from build123d import *

# Parameters (mm, degrees)
Y_KSEKLIK_EKSTR_ZYON1_DEPTH      = 370
Y_KSEKLIK_EKSTR_ZYON2_DEPTH      = 2
Y_KSEKLIK_EKSTR_ZYON2_DEPTH_BACK = 141
KES_EKSTR_ZYON1_DEPTH            = 141


with BuildPart() as part:
    # Çizim1 → Yükseklik-Ekstrüzyon1 (new body)
    with BuildSketch(Plane(origin=(0, 0, 0), x_dir=(0, -1, 0), z_dir=(-1, 0, 0))):
        Polygon((0, 0), (-4, 0), (-4, -4), (-3.5, -4), (-3.5, -0.5), (-0.5, -0.5), (-0.5, -13.15), (-3.5, -13.15), (-3.5, -9.65), (-4, -9.65), (-4, -13.65), (0, -13.65), align=None)
    extrude(amount=-Y_KSEKLIK_EKSTR_ZYON1_DEPTH)

    # Çizim3 → Yükseklik-Ekstrüzyon2 (add, two sides: drawn at the far end of the back side and taken through both)
    with BuildSketch(Plane.ZY.offset(-Y_KSEKLIK_EKSTR_ZYON2_DEPTH_BACK)):
        Polygon((-13.65, 0), (-13.65, 4), (-9.65, 4), (-9.65, 3.5), (-13.15, 3.5), (-13.15, 0.5), (-0.5, 0.5), (-0.5, 3.5), (-4, 3.5), (-4, 4), (0, 4), (0, 0), align=None)
    extrude(amount=Y_KSEKLIK_EKSTR_ZYON2_DEPTH + Y_KSEKLIK_EKSTR_ZYON2_DEPTH_BACK)

    # Çizim5 → Kes-Ekstrüzyon1 (cut)
    with BuildSketch(Plane.ZY.offset(2)):
        Polygon((-13.65, 4), (-13.65, 0), (0, 0), (0, 4), (-4, 4), (-4, 3.5), (-0.5, 3.5), (-0.5, 0.5), (-13.15, 0.5), (-13.15, 3.5), (-9.65, 3.5), (-9.65, 4), align=None)
    extrude(amount=-KES_EKSTR_ZYON1_DEPTH, mode=Mode.SUBTRACT)


solid = part.part
Verification items for the finished model (mm, model axes). A direction names the side the tool comes from. Coordinates: 2 decimals unless noted, no trailing zeros. Order: outer loops, then holes, each group sorted by start corner. A loop starts at its lowest first (then second) coordinate and runs counter-clockwise, first axis right, second up. Notation, with made-up numbers: M -18.5,14.5 L 31.5,14.5 A7 cw 31.5,25.5 Z; hole C 42.5,0.5 d5. An arc over 180 degrees is marked long. Write each question's results on one line, items separated by ' | '.
1) Gauge pin test, flat end, axial feed: pin 1 Ø3 at (x, z) = (255, -4.5) entering from +Y. Record the tip position at first contact, or that the pin passes through.
Solved:
pin 1: stops at y = 4
2) Scan lines: line 1 along Z through (x, y) = (211.5, 0.55); line 2 along Y through (x, z) = (243, -11.75); line 3 along Y through (x, z) = (215, -6.5). Record each from-to range of solid material in increasing order. Write a range as [from, to].
Solved:
line 1: z = [-13.65, -13.15], [-0.5, 0] | line 2: y = [0, 0.5], [3.5, 4] | line 3: y = [0, 0.5]
3) Section check C-C on z = -7.25. Record the cut outline in (x, y).
Solved:
outline: M 139,0 L 370,0 L 370,0.5 L 139,0.5 Z
4) Release check for a two-part mould opening along Y. For faces 3 (the face through (256, 0, -7)), 4 (the face through (256, 4, -12)), 5 (the face through (256, 3.5, -2)), 6 (the face through (370, 0.2, -6.3)) record: pulls with the +Y half, pulls with the -Y half, needs draft (parallel to the pull), parting line crosses it, or undercut.
Solved:
face 3: pulls with the -Y half | face 4: pulls with the +Y half | face 5: undercut | face 6: needs draft
5) Section check B-B on x = 296. Record the cut outline in (y, z).
Solved:
outline: M 0,-13.65 L 4,-13.65 L 4,-9.65 L 3.5,-9.65 L 3.5,-13.15 L 0.5,-13.15 L 0.5,-0.5 L 3.5,-0.5 L 3.5,-4 L 4,-4 L 4,0 L 0,0 Z
6) Access from +Z, -Z, +X, -X, +Y, -Y to the whole of each face (thin tool, end or side, straight path). Record for faces 1 (the face through (256, 2, 0)), 2 (the face through (256, 0.5, -7)).
Solved:
face 1: +Z, +X, -X, +Y, -Y | face 2: +X, -X
7) Section check A-A on y = 2.45. Record the cut outline in (x, z), plus the area to 3 significant figures.
Solved:
outline: M 139,-13.65 L 370,-13.65 L 370,-13.15 L 139,-13.15 Z; M 139,-0.5 L 370,-0.5 L 370,0 L 139,0 Z | area: 231 mm²
